```python
from build123d import *

# Parameters (mm, degrees)
CUT_EXTRUDE1_DEPTH = 15
SKETCH5_OUTSIDE_W  = 38.178
SKETCH5_OUTSIDE_H  = 38.178
CUT_EXTRUDE4_DEPTH = 48.97402978


# Read off the part's stored shape, not the designer's step: Save Bodies1
with BuildPart() as part:
    # Sketch3 → Revolve1 (revolve)
    with BuildSketch(Plane.XY, mode=Mode.PRIVATE) as revolve1_sk:
        Polygon((0, 0), (-4.648047108, 0), (-4.648047108, 0.405570897), (-5.210688758, 0.405570897), (-5.210688758, 0), (-7.649820617, 0), (-10.100522132, 4.244739538), (-10.100522132, 16.176790493), (-7.649820617, 20.42153003), (-4, 20.42153003), (-4, 44.648637254), (0, 44.648637254), align=None)
    revolve(revolve1_sk.sketch.rotate(Axis((0, 44.648637254, 0), (0, -1, 0)), 270), axis=Axis((0, 44.648637254, 0), (0, -1, 0)))

    # Sketch2 → Cut-Extrude1 (cut)
    with BuildSketch(Plane(origin=(0, 0, 0), x_dir=(1, 0, 0), z_dir=(0, 1, 0))):
        Polygon((3.666174209, 0), (1.833087105, 3.175), (-1.833087105, 3.175), (-3.666174209, 0), (-1.833087105, -3.175), (1.833087105, -3.175), align=None)
    extrude(amount=CUT_EXTRUDE1_DEPTH, mode=Mode.SUBTRACT)


with BuildPart() as body_2:
    # Sketch4 → Revolve2 (revolve)
    with BuildSketch(Plane.XY, mode=Mode.PRIVATE) as revolve2_sk:
        with BuildLine():
            Line((10.100522132, 16.176790493), (10.100522132, 4.244739538))
            Line((10.100522132, 4.244739538), (10.600522132, 4.244739538))
            ThreePointArc((10.600522132, 4.244739538), (12.409809018, 10.210765015), (10.600522132, 16.176790493))
            Line((10.600522132, 16.176790493), (10.100522132, 16.176790493))
        make_face()
    revolve(revolve2_sk.sketch.rotate(Axis((0, 44.648637254, 0), (0, -1, 0)), 90), axis=Axis((0, 44.648637254, 0), (0, -1, 0)))

    # Sketch5 outside → Cut-Extrude4 (cut, through all)
    with BuildSketch(Plane(origin=(0, 0, 0), x_dir=(1, 0, 0), z_dir=(0, 1, 0))):
        Rectangle(SKETCH5_OUTSIDE_W, SKETCH5_OUTSIDE_H)
        Polygon((-0.056367181, 11.203062871), (-5.650346846, 9.673953456), (-9.730320636, 5.552716025), (-11.203062871, -0.056367181), (-9.673953456, -5.650346846), (-5.552716025, -9.730320636), (0.056367181, -11.203062871), (5.650346846, -9.673953456), (9.730320636, -5.552716025), (11.203062871, 0.056367181), (9.673953456, 5.650346846), (5.552716025, 9.730320636), align=None, mode=Mode.SUBTRACT)
    extrude(amount=CUT_EXTRUDE4_DEPTH, mode=Mode.SUBTRACT)


solid = part.part
```
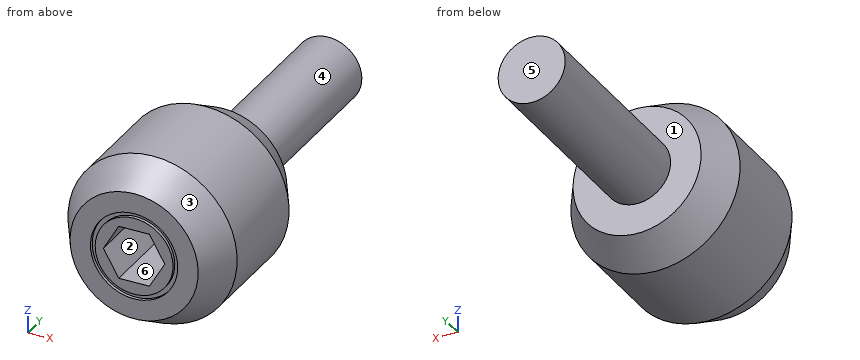
Check sheet for the modelled part. Datum: model origin and axes. Units: mm. Face numbers are marked on the shaded views. A direction names the side the tool comes from. Give positions to 0.01 mm unless a question says otherwise; leave off trailing zeros. Order: outer loops, then holes, each group sorted by start corner. A loop starts at its lowest first (then second) coordinate and runs counter-clockwise, first axis right, second up. Notation, with made-up numbers: (40.25, -23) -> (76.25, -23) arc R17 ccw to (76.25, -18) -> close; hole circle Ø7 at (36, 85.25). An arc over 180 degrees is marked (long way). Use CSV: the item, a comma, the result in double quotes. Start each with the question number.
1) Sectioned sample at A-A, the plane x = 0. Record the boundary of the cut face in (y, z) (3 decimals).
2) Sectioned sample at B-B, the plane y = 3. Record the boundary of the cut face in (x, z) (3 decimals), plus the area to 3 significant figures.
3) Material ranges on line 1 (X direction, y = 0.2, z = 0); line 2 (X direction, y = 0.1, z = 0); line 3 (Y direction, x = -1.25, z = -4), recorded low to high. Write a range as from..to.
4) Go/stop test with flat-tipped pins: P1, Ø1.5, axis at x = 1.5, y = 30, coming from the -Z side; P2, Ø4, axis at x = -3, y = 25, coming from the +Z side; P3, Ø1.5, axis at y = 9, z = 5, coming from the -X side. Record where each tip stops, or that it passes through.
5) Set-up check for the marked faces 4, 5 and 6: record each of +Z, -Z, +X, -X, +Y, -Y from which the full face is reachable in a straight line by a thin tool's end or side.
6) Mould release check, pull along Z, two halves, no side actions. Record for the marked faces 1, 2 and 3: released by +Z, released by -Z, zero draft, split by the parting line, or undercut.
7) Sectioned sample at C-C, the plane y = 33.5. Record the boundary of the cut face in (x, z).
Recorded:
1,outline,"(0, -7.65) -> (4.245, -10.101) -> (16.177, -10.101) -> (20.422, -7.65) -> (20.422, -4) -> (44.649, -4) -> (44.649, 4) -> (20.422, 4) -> (20.422, 7.65) -> (16.177, 10.101) -> (4.245, 10.101) -> (0, 7.65) -> (0, 5.211) -> (0.406, 5.211) -> (0.406, 4.648) -> (0, 4.648) -> (0, 3.175) -> (15, 3.175) -> (15, -3.175) -> (0, -3.175) -> (0, -4.648) -> (0.406, -4.648) -> (0.406, -5.211) -> (0, -5.211) -> close"
2,outline,"circle Ø18.764 at (0, 0); hole (-3.666, 0) -> (-1.833, -3.175) -> (1.833, -3.175) -> (3.666, 0) -> (1.833, 3.175) -> (-1.833, 3.175) -> close"
2,area,"242 mm2"
3,line 1,"-7.77..-5.21, -4.65..-3.67, 3.67..4.65, 5.21..7.77"
3,line 2,"-7.71..-5.21, -4.65..-3.67, 3.67..4.65, 5.21..7.71"
3,line 3,"0..20.42"
4,P1,"z = -3.93"
4,P2,"z = 3.87"
4,P3,"x = -9.16"
5,face 4,"+Y"
5,face 5,"+Z, -Z, +X, -X, +Y"
5,face 6,"-Y"
6,face 1,"zero draft"
6,face 2,"undercut"
6,face 3,"split by the parting line"
7,outline,"circle Ø8 at (0, 0)"
